Answer from the drawing. Dimensions are ordinates in mm from the lowest x, y and z of the part. Give positions to 0.01 mm unless a question says otherwise; leave off trailing zeros. Order: outer loops, then holes, each group sorted by start corner. A loop starts at its lowest first (then second) coordinate and runs counter-clockwise, first axis right, second up. Notation, with made-up numbers: M -16.75,60.25 L 10.25,60.25 A9 cw 10.25,66.25 Z; hole C 37.25,-38 d1. An arc over 180 degrees is marked long. One line per item, written item: value.
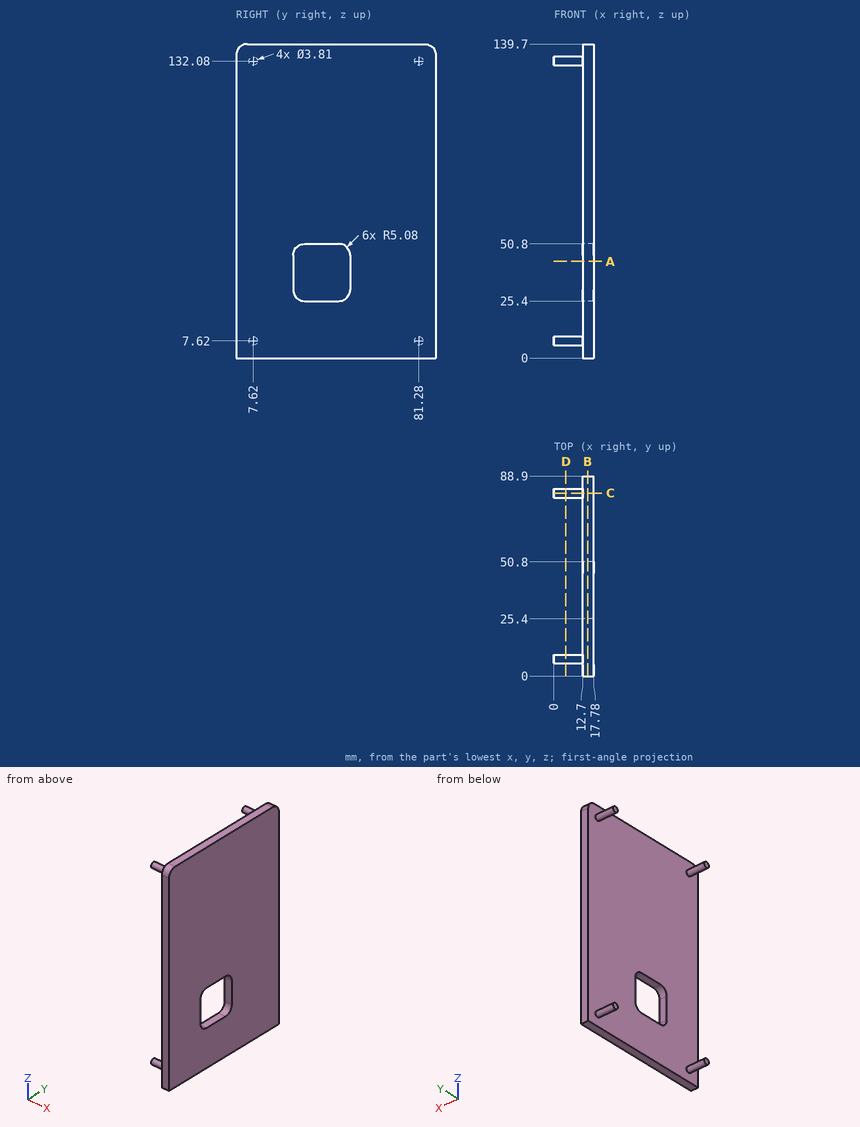
(1) Find the intervals of material crossed by probe 1 along Y at (x, z) = (14.5, 35); probe 2 along Z at (x, y) = (14.75, 41.5); probe 3 along X at (y, z) = (57, 116), in increasing order. Write a range as from..to.
Findings:
probe 1: y = 0..25.4, 50.8..88.9
probe 2: z = 0..25.4, 50.8..139.7
probe 3: x = 12.7..17.78
(2) Section C-C, the plane y = 81.28 is taken. Give the vertices of the cut face in (x, z) (3 decimals).
Findings:
outline: M 0,5.715 L 12.7,5.715 L 12.7,0 L 17.78,0 L 17.78,139.7 L 12.7,139.7 L 12.7,133.985 L 0,133.985 L 0,130.175 L 12.7,130.175 L 12.7,9.525 L 0,9.525 Z
(3) Section A-A, the plane z = 43 is taken. Give the vertices of the cut face in (x, y).
Findings:
outline: M 12.7,0 L 17.78,0 L 17.78,25.4 L 12.7,25.4 Z; M 12.7,50.8 L 17.78,50.8 L 17.78,88.9 L 12.7,88.9 Z
(4) Given P1, Ø6, axis at y = 57.5, z = 70, coming from the -X side; P2, Ø8, axis at x = 5, y = 79, coming from the +Z side (3 decimals), each flat-ended and moving along its own axis, determine where each tip first touches the part or whether it passes through.
Findings:
P1: stops at x = 12.7
P2: stops at z = 133.985
(5) Section D-D, the plane x = 5.25 is taken. Give the vertices of the cut face in (y, z) (3 decimals).
Findings:
outline: C 7.62,7.62 d3.81; C 7.62,132.08 d3.81; C 81.28,7.62 d3.81; C 81.28,132.08 d3.81
(6) Section B-B, the plane x = 15 is taken. Give the vertices of the cut face in (y, z).
Findings:
outline: M 0,0 L 88.9,0 L 88.9,134.62 A5.08 ccw 83.82,139.7 L 5.08,139.7 A5.08 ccw 0,134.62 Z; hole M 25.4,30.48 A5.08 ccw 30.48,25.4 L 45.72,25.4 A5.08 ccw 50.8,30.48 L 50.8,45.72 A5.08 ccw 45.72,50.8 L 30.48,50.8 A5.08 ccw 25.4,45.72 Z
